Autodesk Inventor part; units mm, degrees
ref_plane "YZ Plane" through (0, 0, 0) normal (1, 0, 0) x (0, 1, 0)
ref_plane "XZ Plane" through (0, 0, 0) normal (0, 1, 0) x (-1, 0, 0)
ref_plane "XY Plane" through (0, 0, 0) normal (0, 0, 1) x (1, 0, 0)
sketch "スケッチ1" plane through (0, 0, 0) normal (0, 1, 0) x (-1, 0, 0)
  line L0 (-5, 17.5) -> (5, -17.5) construction
  line L1 (5, 17.5) -> (-5, -17.5) construction
  arc A0 (-5, -12.5) -> (5, -12.5) centre (0, -12.5) ccw
  line L2 (5, 17.5) -> (-5, 17.5)
  line L3 (5, 17.5) -> (5, -12.5)
  line L4 (-5, 17.5) -> (-5, -12.5)
  point P0 (0, 0)
  dimension "d0" = 10
  dimension "d1" = 35
extrude "押し出し1" add sketch "スケッチ1" along normal blind 4
sketch "スケッチ2" plane through (0, 0, 0) normal (0, 1, 0) x (-1, 0, 0)
  arc A0 (-5, -12.5) -> (5, -12.5) centre (0, -12.5) ccw
  circle A1 centre (0, -12.5) radius 3
  point P0 (0, 0)
  dimension "d7" = 6
extrude "押し出し2" cut sketch "スケッチ2" along normal blind 4
sketch "スケッチ3" plane through (0, 0, 0) normal (0, 1, 0) x (-1, 0, 0)
  line L0 (-5, 17.5) -> (5, 17.5)
  line L1 (3, 17.5) -> (3, 12.5)
  line L2 (3, 17.5) -> (8, 17.5) construction
  line L3 (3, 12.5) -> (-3, 12.5)
  line L4 (3, 12.5) -> (9, 12.5) construction
  line L5 (-3, 12.5) -> (-3, 17.5)
  line L6 (-3, 17.5) -> (3, 17.5)
  point P0 (0, 0)
  dimension "d10" = 5
  dimension "d11" = 270
  dimension "d12" = 6
  dimension "d13" = 180
extrude "押し出し3" cut sketch "スケッチ3" along normal blind 4
sketch "スケッチ4" plane through (0, 0, 0) normal (1, 0, 0) x (0, 1, 0)
  circle A0 centre (2, 15.1228) radius 1
  line L0 (0, -12.5) -> (0, 17.5)
  point P0 (0, 0)
  dimension "d16" = 2
  dimension "d18" = 2
extrude "押し出し4" cut sketch "スケッチ4" along normal mid plane 10
properties part number "promo2"
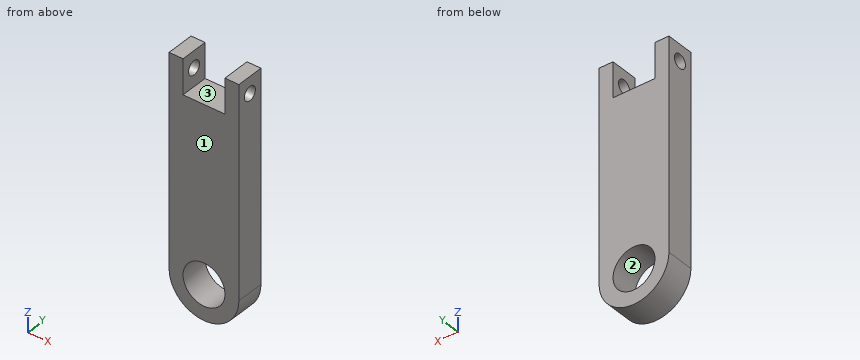
Could you check a few things on this model? Use its own coordinates, in mm. Face numbers are marked on the shaded views. Round coordinates to 2 decimals unless told otherwise and drop trailing zeros. Loops run counter-clockwise (first coordinate to the right, second up) from the corner with the lowest first, then second, coordinate; pieces in that order, holes last. Notation, with made-up numbers: M -33.5,13 L 20.5,13 A24 cw 20.5,27 Z; hole C 60,68 d4. An arc over 180 degrees is marked long. Put each result on its own line as item: value.
Q1. For pin 1 (1.2 mm diameter, centred on x = 1, y = 2.5, fed in from +Z), with a flat end and sliding along its axis, tell me the tip position at first contact or that it passes through.
Check result:
pin 1: z = 12.5
Q2. Imagine slicing it at D-D (x = -2). Write out the boundary of the cut face in (y, z).
Check result:
outline: M 0,-17.08 L 4,-17.08 L 4,-14.74 L 0,-14.74 Z; M 0,-10.26 L 4,-10.26 L 4,12.5 L 0,12.5 Z
Q3. Imagine slicing it at A-A (y = 2). Write out the boundary of the cut face in (x, z).
Check result:
outline: M -5,-12.5 A5 ccw 5,-12.5 L 5,14.12 L 3,14.12 L 3,12.5 L -3,12.5 L -3,14.12 L -5,14.12 Z; M -5,16.12 L -3,16.12 L -3,17.5 L -5,17.5 Z; M 3,16.12 L 5,16.12 L 5,17.5 L 3,17.5 Z; hole C 0,-12.5 d6
Q4. Imagine slicing it at B-B (x = 0). Write out the boundary of the cut face in (y, z), then the cut area to 3 significant figures.
Check result:
outline: M 0,-17.5 L 4,-17.5 L 4,-15.5 L 0,-15.5 Z; M 0,-9.5 L 4,-9.5 L 4,12.5 L 0,12.5 Z
area: 96.0 mm2
Q5. Imagine slicing it at C-C (y = 3.65). Write out the boundary of the cut face in (x, z), then the cut area to 3 significant figures.
Check result:
outline: M -5,-12.5 A5 ccw 5,-12.5 L 5,17.5 L 3,17.5 L 3,12.5 L -3,12.5 L -3,17.5 L -5,17.5 Z; hole C 0,-12.5 d6
area: 281 mm2
Q6. I need wall thicknesses on probe 1 along Z at (x, y) = (0, 1.1); probe 2 along Z at (x, y) = (3.75, 2.1); probe 3 along X at (y, z) = (3.3, -10.5). Which ranges of each line are inside material? Lowest first, please.
Check result:
probe 1: -17.5 to -15.5, -9.5 to 12.5
probe 2: -15.81 to 14.13, 16.12 to 17.5
probe 3: -5 to -2.24, 2.24 to 5
Q7. Thinking about a two-plate mould opening in Z: for the marked faces 1, 2 and 3, which applies, released by +Z, released by -Z, zero draft, split by the parting line, or undercut?
Check result:
face 1: zero draft
face 2: undercut
face 3: released by +Z
